Part model, mm, in its own coordinate system. A direction names the side the tool comes from. Give positions to 0.01 mm unless a question says otherwise; leave off trailing zeros. Write each loop counter-clockwise with the first axis right and the second up, starting at its lowest first coordinate (ties: lowest second). Pieces come first, ordered by that corner, then holes. Notation, with made-up numbers: M -26,83.5 L 1,83.5 A27 ccw 1,105.5 Z; hole C 17,40.5 d9. An arc over 180 degrees is marked long. Use CSV: the item, a comma, the result in double quotes. Start each with the question number.
1. Band-saw the part on C-C, the plane z = -6.5. List the corners of the cut face in (x, y).
2. Band-saw the part on A-A, the plane y = 0.55. Count the separate pieces of the cut face and the enclosed holes in it, then the cut area to 3 significant figures.
3. Mould opens along X. For faces 4 (the face through (-1.352, -1.268, 4.292)), 5 (the face through (2, -2.5, 2)), 6 (the face through (1.4, 0, -1.4)) say: pulls with the +X half, pulls with the -X half, needs draft (parallel to the pull), parting line crosses it, or undercut.
4. Drill centre lines: line 1 along Z through (x, y) = (7.75, 1.7); line 2 along Y through (x, z) = (1.25, 6.75); line 3 along Z through (x, y) = (2, -0.45). Where is each one in solid material? Low to high. Write a range as from..to.
5. Band-saw the part on B-B, the plane x = -8.75. List the corners of the cut face in (y, z), then the cut area to 3 significant figures.
6. Band-saw the part on D-D, the plane x = 4.75. List the corners of the cut face in (y, z).
7. 3-axis set-ups, long thin cutter, end or side, ignore diameter. For faces 1 (the face through (0, 1.2, 2)), 2 (the face through (3.2, 1, 10)), 3 (the face through (0, 0, 5)): which of +Z, -Z, +X, -X, +Y, -Y reach the whole face in a straight line?
8. Drop flat-ended pins along their axis: pin 1 Ø2 at (x, y) = (-2, 1.5) entering from +Z; pin 2 Ø4 at (x, z) = (0, 0) entering from -Y; pin 3 Ø2 at (y, z) = (-0.5, -2.5) entering from +X. Give the stop position or say it passes through.
from build123d import *

# Parameters (mm, degrees)
SKETCH1_R           = 10.5
SKETCH1_R_2         = 1.5
SKETCH1_R_3         = 0.5
BOSS_EXTRUDE1_DEPTH = 2
SKETCH2_R           = 4.5
SKETCH2_R_2         = 3.5
BOSS_EXTRUDE2_DEPTH = 0.5
CUT_EXTRUDE1_START  = -0.8
SKETCH3_R           = 3.5
SKETCH3_R_2         = 1.5
CUT_EXTRUDE1_DEPTH  = 0.8
BOSS_EXTRUDE3_START = 2.5
SKETCH4_R           = 4.5
SKETCH4_R_2         = 2.5
BOSS_EXTRUDE3_DEPTH = 2.5
CUT_EXTRUDE3_DEPTH  = 2.5


with BuildPart() as part:
    # Sketch1 → Boss-Extrude1 (new body)
    with BuildSketch(Plane(origin=(0, 0, 0), x_dir=(1, 0, 0), z_dir=(0, 1, 0))):
        with Locations(Location((0, 0, 0), (0, 0, 270))):
            Circle(SKETCH1_R)
        with Locations(Location((0, 0, 0), (0, 0, 270))):
            Circle(SKETCH1_R_2, mode=Mode.SUBTRACT)
        with Locations(Location((2.907171218, 7.987387277, 0), (0, 0, 270))):
            Circle(SKETCH1_R_3, mode=Mode.SUBTRACT)
        with Locations(Location((-2.907171218, 7.987387277, 0), (0, 0, 270))):
            Circle(SKETCH1_R_3, mode=Mode.SUBTRACT)
        with Locations(Location((2.907171218, -7.987387277, 0), (0, 0, 90))):
            Circle(SKETCH1_R_3, mode=Mode.SUBTRACT)
        with Locations(Location((-2.907171218, -7.987387277, 0), (0, 0, 90))):
            Circle(SKETCH1_R_3, mode=Mode.SUBTRACT)
        with Locations(Location((0, -8.5, 0), (0, 0, 90))):
            Circle(SKETCH1_R_3, mode=Mode.SUBTRACT)
        with Locations(Location((8.5, 0, 0), (0, 0, 270))):
            Circle(SKETCH1_R_3, mode=Mode.SUBTRACT)
        with Locations(Location((7.987387277, 2.907171218, 0), (0, 0, 270))):
            Circle(SKETCH1_R_3, mode=Mode.SUBTRACT)
        with Locations(Location((7.987387277, -2.907171218, 0), (0, 0, 270))):
            Circle(SKETCH1_R_3, mode=Mode.SUBTRACT)
        with Locations(Location((-7.987387277, -2.907171218, 0), (0, 0, 90))):
            Circle(SKETCH1_R_3, mode=Mode.SUBTRACT)
        with Locations(Location((-8.5, 0, 0), (0, 0, 90))):
            Circle(SKETCH1_R_3, mode=Mode.SUBTRACT)
        with Locations(Location((-7.987387277, 2.907171218, 0), (0, 0, 90))):
            Circle(SKETCH1_R_3, mode=Mode.SUBTRACT)
        with Locations(Location((0, 8.5, 0), (0, 0, 270))):
            Circle(SKETCH1_R_3, mode=Mode.SUBTRACT)
    extrude(amount=BOSS_EXTRUDE1_DEPTH)

    # Sketch2 → Boss-Extrude2 (add)
    with BuildSketch(Plane(origin=(0, 2, 0), x_dir=(1, 0, 0), z_dir=(0, 1, 0))):
        with Locations(Location((0, 0, 0), (0, 0, 270))):
            Circle(SKETCH2_R)
        with Locations(Location((0, 0, 0), (0, 0, 270))):
            Circle(SKETCH2_R_2, mode=Mode.SUBTRACT)
    extrude(amount=BOSS_EXTRUDE2_DEPTH)

    # Sketch3 → Cut-Extrude1 (cut)
    with BuildSketch(Plane(origin=(0, 2, 0), x_dir=(1, 0, 0), z_dir=(0, 1, 0)).offset(CUT_EXTRUDE1_START)):
        with Locations(Location((0, 0, 0), (0, 0, 270))):
            Circle(SKETCH3_R)
        with Locations(Location((0, 0, 0), (0, 0, 270))):
            Circle(SKETCH3_R_2, mode=Mode.SUBTRACT)
    extrude(amount=CUT_EXTRUDE1_DEPTH, mode=Mode.SUBTRACT)

    # Sketch4 → Boss-Extrude3 (add)
    with BuildSketch(Plane.XZ.offset(BOSS_EXTRUDE3_START)):
        with Locations(Location((0, 0, 0), (0, 0, 90))):
            Circle(SKETCH4_R)
        with Locations(Location((0, 0, 0), (0, 0, 270))):
            Circle(SKETCH4_R_2, mode=Mode.SUBTRACT)
    extrude(amount=-BOSS_EXTRUDE3_DEPTH)

    # Sketch5 → Cut-Extrude3 (cut)
    with BuildSketch(Plane.XZ.offset(2.5)):
        with BuildLine():
            Line((0.299038106, 2.482050808), (0, 3))
            Line((0, 3), (-0.299038106, 2.482050808))
            ThreePointArc((-0.299038106, 2.482050808), (-0.391086163, 2.469220851), (-0.482593741, 2.452978451))
            Line((-0.482593741, 2.452978451), (-0.927050983, 2.853169549))
            Line((-0.927050983, 2.853169549), (-1.051398019, 2.268162738))
            ThreePointArc((-1.051398019, 2.268162738), (-1.134976249, 2.22751631), (-1.216985951, 2.183791473))
            Line((-1.216985951, 2.183791473), (-1.763355757, 2.427050983))
            Line((-1.763355757, 2.427050983), (-1.70083977, 1.832251096))
            ThreePointArc((-1.70083977, 1.832251096), (-1.767766953, 1.767766953), (-1.832251096, 1.70083977))
            Line((-1.832251096, 1.70083977), (-2.427050983, 1.763355757))
            Line((-2.427050983, 1.763355757), (-2.183791473, 1.216985951))
            ThreePointArc((-2.183791473, 1.216985951), (-2.22751631, 1.134976249), (-2.268162738, 1.051398019))
            Line((-2.268162738, 1.051398019), (-2.853169549, 0.927050983))
            Line((-2.853169549, 0.927050983), (-2.452978451, 0.482593741))
            ThreePointArc((-2.452978451, 0.482593741), (-2.469220851, 0.391086163), (-2.482050808, 0.299038106))
            Line((-2.482050808, 0.299038106), (-3, 0))
            Line((-3, 0), (-2.482050808, -0.299038106))
            ThreePointArc((-2.482050808, -0.299038106), (-2.469220851, -0.391086163), (-2.452978451, -0.482593741))
            Line((-2.452978451, -0.482593741), (-2.853169549, -0.927050983))
            Line((-2.853169549, -0.927050983), (-2.268162738, -1.051398019))
            ThreePointArc((-2.268162738, -1.051398019), (-2.22751631, -1.134976249), (-2.183791473, -1.216985951))
            Line((-2.183791473, -1.216985951), (-2.427050983, -1.763355757))
            Line((-2.427050983, -1.763355757), (-1.832251096, -1.70083977))
            ThreePointArc((-1.832251096, -1.70083977), (-1.767766953, -1.767766953), (-1.70083977, -1.832251096))
            Line((-1.70083977, -1.832251096), (-1.763355757, -2.427050983))
            Line((-1.763355757, -2.427050983), (-1.216985951, -2.183791473))
            ThreePointArc((-1.216985951, -2.183791473), (-1.134976249, -2.22751631), (-1.051398019, -2.268162738))
            Line((-1.051398019, -2.268162738), (-0.927050983, -2.853169549))
            Line((-0.927050983, -2.853169549), (-0.482593741, -2.452978451))
            ThreePointArc((-0.482593741, -2.452978451), (-0.391086163, -2.469220851), (-0.299038106, -2.482050808))
            Line((-0.299038106, -2.482050808), (0, -3))
            Line((0, -3), (0.299038106, -2.482050808))
            ThreePointArc((0.299038106, -2.482050808), (0.391086163, -2.469220851), (0.482593741, -2.452978451))
            Line((0.482593741, -2.452978451), (0.927050983, -2.853169549))
            Line((0.927050983, -2.853169549), (1.051398019, -2.268162738))
            ThreePointArc((1.051398019, -2.268162738), (1.134976249, -2.22751631), (1.216985951, -2.183791473))
            Line((1.216985951, -2.183791473), (1.763355757, -2.427050983))
            Line((1.763355757, -2.427050983), (1.70083977, -1.832251096))
            ThreePointArc((1.70083977, -1.832251096), (1.767766953, -1.767766953), (1.832251096, -1.70083977))
            Line((1.832251096, -1.70083977), (2.427050983, -1.763355757))
            Line((2.427050983, -1.763355757), (2.183791473, -1.216985951))
            ThreePointArc((2.183791473, -1.216985951), (2.22751631, -1.134976249), (2.268162738, -1.051398019))
            Line((2.268162738, -1.051398019), (2.853169549, -0.927050983))
            Line((2.853169549, -0.927050983), (2.452978451, -0.482593741))
            ThreePointArc((2.452978451, -0.482593741), (2.469220851, -0.391086163), (2.482050808, -0.299038106))
            Line((2.482050808, -0.299038106), (3, 0))
            Line((3, 0), (2.482050808, 0.299038106))
            ThreePointArc((2.482050808, 0.299038106), (2.469220851, 0.391086163), (2.452978451, 0.482593741))
            Line((2.452978451, 0.482593741), (2.853169549, 0.927050983))
            Line((2.853169549, 0.927050983), (2.268162738, 1.051398019))
            ThreePointArc((2.268162738, 1.051398019), (2.22751631, 1.134976249), (2.183791473, 1.216985951))
            Line((2.183791473, 1.216985951), (2.427050983, 1.763355757))
            Line((2.427050983, 1.763355757), (1.832251096, 1.70083977))
            ThreePointArc((1.832251096, 1.70083977), (1.767766953, 1.767766953), (1.70083977, 1.832251096))
            Line((1.70083977, 1.832251096), (1.763355757, 2.427050983))
            Line((1.763355757, 2.427050983), (1.216985951, 2.183791473))
            ThreePointArc((1.216985951, 2.183791473), (1.134976249, 2.22751631), (1.051398019, 2.268162738))
            Line((1.051398019, 2.268162738), (0.927050983, 2.853169549))
            Line((0.927050983, 2.853169549), (0.482593741, 2.452978451))
            ThreePointArc((0.482593741, 2.452978451), (0.391086163, 2.469220851), (0.299038106, 2.482050808))
        make_face()
    extrude(amount=-CUT_EXTRUDE3_DEPTH, mode=Mode.SUBTRACT)


solid = part.part
Output:
1,outline,"M -8.25,0 L 8.25,0 L 8.25,2 L -8.25,2 Z"
2,separate pieces,"1"
2,enclosed holes,"13"
2,area,"330 mm²"
3,face 4,"parting line crosses it"
3,face 5,"needs draft"
3,face 6,"undercut"
4,line 1,"z = -7.08..-3.35, -2.47..2.47, 3.35..7.08"
4,line 2,"y = 0..2"
4,line 3,"z = -4.03..-1.72, 1.72..4.03"
5,outline,"M 0,-5.8 L 2,-5.8 L 2,-0.43 L 0,-0.43 Z; M 0,0.43 L 2,0.43 L 2,5.8 L 0,5.8 Z"
5,area,"21.5 mm²"
6,outline,"M 0,-9.36 L 2,-9.36 L 2,9.36 L 0,9.36 Z"
7,face 1,"+Y"
7,face 2,"+Y, -Y"
7,face 3,"-Y"
8,pin 1,"stops at z = 10.45"
8,pin 2,"stops at y = 0"
8,pin 3,"stops at x = 10.37"
